Here's how the part is built. I have some questions about the finished solid (model axes, mm). A direction names the side the tool comes from. Coordinates: 2 decimals unless noted, no trailing zeros. Loops run counter-clockwise (first coordinate to the right, second up) from the corner with the lowest first, then second, coordinate; pieces in that order, holes last. Notation, with made-up numbers: (-22.5, 40) -> (-14.5, 40) arc R12 cw to (-14.5, 44) -> close; hole circle Ø4 at (30.5, 22). An arc over 180 degrees is marked (long way). Use CSV: the item, a comma, the result in double quotes. Start each with the question number.
from build123d import *

# Parameters (mm, degrees)
F0_R     = 12.7
F1_DEPTH = 3.81
F2_W     = 3.0322148232
F2_H     = 2.8683111304
F3_DEPTH = 19.05
F4_W     = 5.6596440263
F4_H     = 2.8683111304
F4_W_2   = 3.0322148232
F4_W_3   = 5.5680392543
F5_DEPTH = 2.54
F6_W     = 3.0350781744
F6_H     = 2.8683111304
F7_DEPTH = 6.35


with BuildPart() as f1:
    # F0 (on Top) → F1 (new body)
    with BuildSketch(Plane.XY):
        Circle(F0_R)
    extrude(amount=F1_DEPTH)

    # F2 (on face) → F3 (join)
    with BuildSketch(Plane.XY.offset(3.81)):
        with Locations((-0.1229271875, -0.2458557137)):
            Rectangle(F2_W, F2_H)
    extrude(amount=F3_DEPTH)

    # F4 (on face) → F5 (join)
    with BuildSketch(Plane.XY.offset(22.86)):
        with Locations((-4.4688566122, -0.2458557137)):
            Rectangle(F4_W, F4_H)
        with Locations((-0.1229271875, -0.2458557137)):
            Rectangle(F4_W_2, F4_H)
        with Locations((4.1771998513, -0.2458557137)):
            Rectangle(F4_W_3, F4_H)
    extrude(amount=F5_DEPTH)

    # F6 (on face) → F7 (join)
    with BuildSketch(Plane.XY.offset(25.4)):
        with Locations((-0.1373158884, -0.2458557137)):
            Rectangle(F6_W, F6_H)
    extrude(amount=F7_DEPTH)


solid = f1.part
1) For P1, Ø10, axis at x = 6, z = 12.5, coming from the +Y side; P2, Ø2.5, axis at y = 0, z = 16, coming from the +X side; P3, Ø0.9, axis at x = 3, y = -0.5, coming from the +Z side, each with a flat end and sliding along its axis, tell me the tip position at first contact or that it passes through.
2) Thinking about a two-plate mould opening in Z: for faces 5 (the face through (0, 0, 0)), 6 (the face through (4, 0, 25.4)), 7 (the face through (1.393, 0, 13)), 8 (the face through (-1.655, 0, 29)), which applies, pulls with the +Z half, pulls with the -Z half, needs draft (parallel to the pull), parting line crosses it, or undercut?
3) I want a section at D-D, the plane z = 9.5. Please give me the cut outline in (x, y), plus the area to 3 significant figures.
4) Which directions (+Z, -Z, +X, -X, +Y, -Y) give clear straight access to the entire face, cutting with the end or side of a thin tool? Please do faces 1 (the face through (-1.639, 0, 13)), 2 (the face through (4, 0, 22.86)), 3 (the face through (-7.299, 0, 24)), 4 (the face through (1.38, 0, 29)).
5) I want a section at A-A, the plane x = -4.25. Please give me the cut outline in (y, z), plus the area to 3 significant figures.
6) Please list where these lines run through material, in increasing order: L1, parallel to Z at x = 7, y = -1; L2, parallel to X at y = 1, z = 14; L3, parallel to Y at x = 0.5, z = 22.5. Write a range as [from, to].
7) I want a section at B-B, the plane y = 0. Please give me the cut outline in (x, z), plus the area to 3 significant figures.
8) I want a section at C-C, the plane x = 0. Please give me the cut outline in (y, z).
Return value:
1,P1,"stops at y = 1.19"
1,P2,"stops at x = 1.39"
1,P3,"stops at z = 25.4"
2,face 5,"pulls with the -Z half"
2,face 6,"pulls with the +Z half"
2,face 7,"undercut"
2,face 8,"needs draft"
3,outline,"(-1.64, -1.68) -> (1.39, -1.68) -> (1.39, 1.19) -> (-1.64, 1.19) -> close"
3,area,"8.70 mm²"
4,face 1,"-X, +Y, -Y"
4,face 2,"+X, +Y, -Y"
4,face 3,"+Z, -X, +Y, -Y"
4,face 4,"+Z, +X, +Y, -Y"
5,outline,"(-11.97, 0) -> (11.97, 0) -> (11.97, 3.81) -> (-11.97, 3.81) -> close; (-1.68, 22.86) -> (1.19, 22.86) -> (1.19, 25.4) -> (-1.68, 25.4) -> close"
5,area,"98.5 mm²"
6,L1,"z = [0, 3.81]"
6,L2,"x = [-1.64, 1.39]"
6,L3,"y = [-1.68, 1.19]"
7,outline,"(-12.7, 0) -> (12.7, 0) -> (12.7, 3.81) -> (1.39, 3.81) -> (1.39, 22.86) -> (6.96, 22.86) -> (6.96, 25.4) -> (1.38, 25.4) -> (1.38, 31.75) -> (-1.65, 31.75) -> (-1.65, 25.4) -> (-7.3, 25.4) -> (-7.3, 22.86) -> (-1.64, 22.86) -> (-1.64, 3.81) -> (-12.7, 3.81) -> close"
7,area,"210 mm²"
8,outline,"(-12.7, 0) -> (12.7, 0) -> (12.7, 3.81) -> (1.19, 3.81) -> (1.19, 31.75) -> (-1.68, 31.75) -> (-1.68, 3.81) -> (-12.7, 3.81) -> close"
